Read the model definition and answer for the solid it produces. Units are mm, in the model's axes. A direction names the side the tool comes from. Give positions to 0.01 mm unless a question says otherwise; leave off trailing zeros. Write each loop counter-clockwise with the first axis right and the second up, starting at its lowest first coordinate (ties: lowest second). Pieces come first, ordered by that corner, then holes.
```python
from build123d import *

# Parameters (mm, degrees)
SKETCH_1_R               = 22.25
SKETCH_1_R_2             = 21.05
EXTRUDE_1_DEPTH          = 41
SKETCH_2_R               = 22.25
SKETCH_2_R_2             = 13.05
EXTRUDE_2_DEPTH          = 1.5
SKETCH_3_R               = 28.25
SKETCH_3_R_2             = 21.05
EXTRUDE_3_DEPTH          = 4
SKETCH_4_R               = 23.25
SKETCH_4_R_2             = 22.25
EXTRUDE_4_DEPTH          = 6
SKETCH_5_R               = 22.5
SKETCH_5_R_2             = 22.25
EXTRUDE_5_DEPTH          = 7
SKETCH_6_R               = 2
CUT_EXTRUDE_1_DEPTH      = 7
PATTERN_CIRCULAR_1_COUNT = 6
CHAMFER_1_SIZE           = 0.5


with BuildPart() as part:
    # 草图1 → 凸台-拉伸1 (new body)
    with BuildSketch(Plane.XY):
        Circle(SKETCH_1_R)
        Circle(SKETCH_1_R_2, mode=Mode.SUBTRACT)
    extrude(amount=EXTRUDE_1_DEPTH)

    # 草图2 → 凸台-拉伸2 (add)
    with BuildSketch(Plane.XY.offset(41)):
        Circle(SKETCH_2_R)
        Circle(SKETCH_2_R_2, mode=Mode.SUBTRACT)
    extrude(amount=-EXTRUDE_2_DEPTH)

    # 草图3 → 凸台-拉伸3 (add)
    with BuildSketch(Plane(origin=(0, 0, 0), x_dir=(-1, 0, 0), z_dir=(0, 0, -1))):
        Circle(SKETCH_3_R)
        Circle(SKETCH_3_R_2, mode=Mode.SUBTRACT)
    extrude(amount=-EXTRUDE_3_DEPTH)

    # 草图4 → 凸台-拉伸4 (add)
    with BuildSketch(Plane.XY.offset(4)):
        Circle(SKETCH_4_R)
        Circle(SKETCH_4_R_2, mode=Mode.SUBTRACT)
    extrude(amount=EXTRUDE_4_DEPTH)

    # 草图5 → 凸台-拉伸5 (add)
    with BuildSketch(Plane.XY.offset(10)):
        Circle(SKETCH_5_R)
        Circle(SKETCH_5_R_2, mode=Mode.SUBTRACT)
    extrude(amount=EXTRUDE_5_DEPTH)

    # 草图6 → 切除-拉伸1 (cut)
    with BuildSketch(Plane(origin=(0, 0, 39.5), x_dir=(-1, 0, 0), z_dir=(0, 0, -1))):
        with Locations((12.374368671, 12.374368671)):
            Circle(SKETCH_6_R)
        with Locations((17.5, 0)):
            Circle(SKETCH_6_R)
        with Locations((12.374368671, -12.374368671)):
            Circle(SKETCH_6_R)
        with Locations((0, -17.5)):
            Circle(SKETCH_6_R)
        with Locations((-12.374368671, -12.374368671)):
            Circle(SKETCH_6_R)
        with Locations((-17.5, 0)):
            Circle(SKETCH_6_R)
        with Locations((-12.374368671, 12.374368671)):
            Circle(SKETCH_6_R)
        with Locations((0, 17.5)):
            Circle(SKETCH_6_R)
    extrude(amount=-CUT_EXTRUDE_1_DEPTH, mode=Mode.SUBTRACT)

    # 草图9 → M4 螺纹孔1 (revolve, cut)
    with BuildSketch(Plane(origin=(0, 25.5, 4), x_dir=(0, -1, 0), z_dir=(1, 0, 0))):
        Polygon((0, 0), (0, 11.091420021), (1.65, 10.1), (1.65, 0), align=None)
    hole_wizard_m4_1 = revolve(axis=Axis((0, 25.5, 10.35), (0, 0, -1)), mode=Mode.SUBTRACT)

    # 阵列(圆周)1: M4 螺纹孔1 ×6 about axis
    pattern_circular_1_axis = Axis((0, 0, 0), (0, 0, 1))
    for i in range(1, PATTERN_CIRCULAR_1_COUNT):
        add(hole_wizard_m4_1.rotate(pattern_circular_1_axis, i * 360 / PATTERN_CIRCULAR_1_COUNT), mode=Mode.SUBTRACT)

    # 倒角1
    chamfer_1_edges = [part.edges().sort_by_distance(p)[0] for p in [
        (28.25, 0, 4),
        (28.25, 0, 0),
        (-22.25, 0, 41),
        (-21.05, 0, 0),
    ]]
    chamfer(chamfer_1_edges, length=CHAMFER_1_SIZE)


solid = part.part
```
Item 1: Find the intervals of material crossed by line 1 along Y through (x, z) = (0, 40.4); line 2 along Z through (x, y) = (-7, 15); line 3 along Y through (x, z) = (17.5, 40.3), in increasing order.
Result set:
line 1: y = -22.25 to -19.5, -15.5 to -13.05, 13.05 to 15.5, 19.5 to 22.25
line 2: z = 39.5 to 41
line 3: y = -13.74 to -2, 2 to 13.74
Item 2: Section B-B (y = 0) is taken. Give the number of separate pieces and of enclosed holes in the cut face, and give its area (3 significant figures).
Result set:
separate pieces: 4
enclosed holes: 0
area: 173 mm2
Item 3: Section D-D (z = 35.5) is taken. Write down the section's boundary in (x, y), and give its area (3 significant figures).
Result set:
outline: circle Ø44.5 at (0, 0); hole circle Ø42.1 at (0, 0)
area: 163 mm2
Item 4: Which of the six approach directions +Z, -Z, +X, -X, +Y, -Y give full straight-line access (tool end or side, diameter ignored) to faces 4 (the cylindrical face through (13.962, -13.591, 40.24)), 5 (the flat face through (-12.2, 19.1, 10)), 6 (the flat face through (-10, -9, 39.5))?
Result set:
face 4: +Z, -Z
face 5: +Z
face 6: -Z
Item 5: Determine the mould class of faces 1 (the flat face through (6, 21, 0)), 2 (the cylindrical face through (-15.9, -1.2, 40.2)), 3 (the cylindrical face through (22.176, 6.984, 6.958)) for opening direction X: pulls with the +X half, pulls with the -X half, needs draft (parallel to the pull), parting line crosses it, or undercut.
Result set:
face 1: needs draft
face 2: undercut
face 3: parting line crosses it
Item 6: Section A-A (z = 6.5) is taken. Write down the section's boundary in (x, y), and give its area (3 significant figures).
Result set:
outline: circle Ø46.5 at (0, 0); hole circle Ø42.1 at (0, 0)
area: 306 mm2
Item 7: Each of these flat-tipped pins is pushed along its axis until it touches: pin 1 Ø3.5 at (x, y) = (-12.37, -12.37) entering from -Z; pin 2 Ø4 at (x, z) = (22, 19.5) entering from +Y; pin 3 Ø4 at (x, z) = (10.5, 25.5) entering from -Y; pin 4 Ø2 at (x, z) = (-12, 9) entering from +Y. Where does it stop, or does it pass through?
Result set:
pin 1: passes through
pin 2: stops at y = 9.75
pin 3: stops at y = -20.56
pin 4: stops at y = 20.48
